For this review, use the dimensioned drawing (mm, ordinates from the lowest corner) and the shaded views. A direction names the side the tool comes from. Round coordinates to 2 decimals unless told otherwise and drop trailing zeros. Write each loop counter-clockwise with the first axis right and the second up, starting at its lowest first coordinate (ties: lowest second). Pieces come first, ordered by that corner, then holes. Notation, with made-up numbers: M 29.5,-30.5 L 77.5,-30.5 A25 cw 77.5,-13.5 Z; hole C -14.75,-32 d11. An arc over 180 degrees is marked long. Use CSV: the item, a comma, the result in double quotes.
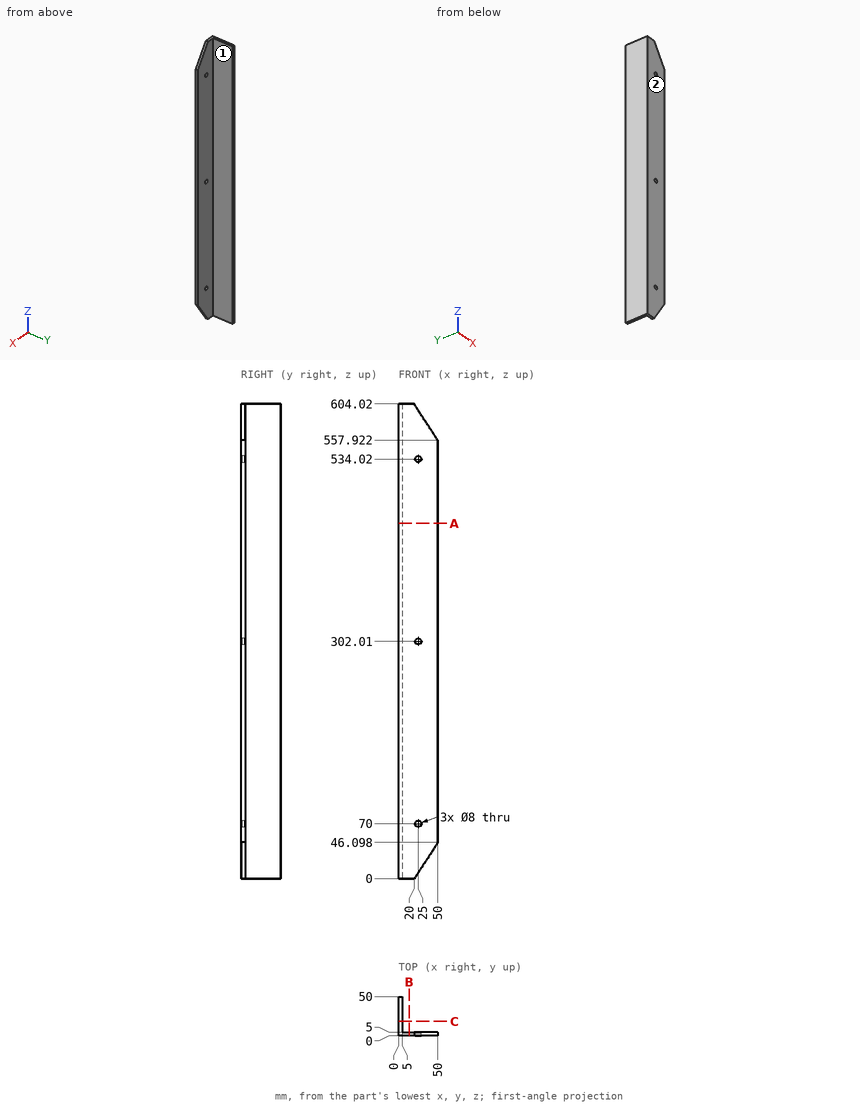
1) Machinability: for the marked faces 1 and 2, which of the approach directions +Z, -Z, +X, -X, +Y, -Y give a long, thin tool a straight path to every point of the face, cutting with its end or side? Answer none if there is none.
Answers:
face 1,"+Z, -Z, +X, +Y"
face 2,"+Z, -Z, +X, -X, -Y"
2) Add section A-A on z = 452. Write out the cut boundary in (x, y), then the cut area to 3 significant figures.
Answers:
outline,"M 0,0 L 50,0 L 50,5 L 5,5 L 5,50 L 0,50 Z"
area,"475 mm²"
3) For pin 1 Ø22.5 at (y, z) = (18, 203) entering from +X; pin 2 Ø6 at (x, z) = (43, 473.5) entering from +Y, all flat-tipped, find the tip position at first contact; note any pin that passes through.
Answers:
pin 1,"x = 5"
pin 2,"y = 5"
4) Wall thickness on line 1 along X through (y, z) = (3, 302); line 2 along X through (y, z) = (22.5, 243.5): over which ranges is each line inside the solid? List them lowest first. Write a range as [from, to].
Answers:
line 1,"[0, 21], [29, 50]"
line 2,"[0, 5]"
5) Add section B-B on x = 13.5. Write out the cut boundary in (y, z), then the cut area to 3 significant figures.
Answers:
outline,"M 0,0 L 5,0 L 5,604.02 L 0,604.02 Z"
area,"3,020 mm²"
